Check sheet for the modelled part. Datum: model origin and axes. Units: mm. Face numbers are marked on the shaded views. A direction names the side the tool comes from. Coordinates: 2 decimals unless noted, no trailing zeros. Write each loop counter-clockwise with the first axis right and the second up, starting at its lowest first coordinate (ties: lowest second). Pieces come first, ordered by that corner, then holes. Notation, with made-up numbers: M 85.25,-26.5 L 109.25,-26.5 A35 ccw 109.25,6.5 Z; hole C 88.25,-33 d5. An arc over 180 degrees is marked long. Answer as CSV lines item,"result". Start each with the question number.
Q1. Depth check by flat-ended pin: pin 1 Ø15 at (x, y) = (31.5, -6.5) entering from +Z; pin 2 Ø5 at (y, z) = (-14, 23.5) entering from +X; pin 3 Ø5.5 at (x, z) = (30.5, 9.5) entering from -Y. Enter the tip coordinate at first touch or a pass-through.
Q2. Sectioned sample at B-B, the plane z = 14.5. Record the cut outline in (x, y), then the cut area to 3 significant figures.
Q3. Sectioned sample at C-C, the plane x = 34. Record the cut outline in (y, z).
Q4. Sectioned sample at A-A, the plane y = -9. Record the cut outline in (x, z), then the cut area to 3 significant figures.
Q5. Access from +Z, -Z, +X, -X, +Y, -Y to the whole of each face (thin tool, end or side, straight path). Record for the marked faces 1, 2, 3 and 4.
Q6. Sectioned sample at D-D, the plane x = 16.5. Record the cut outline in (y, z).
Q7. Thickness scan on line 1 along X through (y, z) = (-27.5, 12); line 2 along X through (y, z) = (-17, 25). Record the ranges inside material, lowest first. Write a range as from..to.
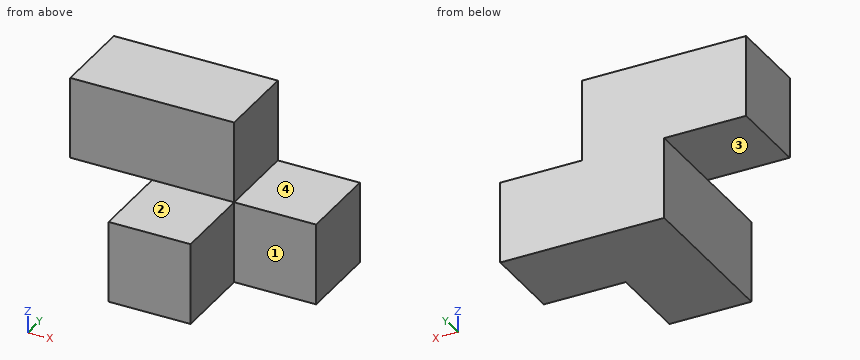
from build123d import *

# Parameters (mm, degrees)
F1_DEPTH = 19.05
F2_W     = 19.05
F2_H     = 19.05
F3_DEPTH = 19.05


with BuildPart() as f1:
    # F0 (on Front) → F1 (new body)
    with BuildSketch(Plane.XZ):
        Polygon((0, 19.05), (0, 0), (38.1, 0), (38.1, 19.05), (19.05, 19.05), (19.05, 38.1), (-19.05, 38.1), (-19.05, 19.05), align=None)
    extrude(amount=F1_DEPTH)

    # F2 (on face) → F3 (join)
    with BuildSketch(Plane.XZ.offset(19.05)):
        with Locations((9.525, 9.525)):
            Rectangle(F2_W, F2_H)
    extrude(amount=F3_DEPTH)


solid = f1.part
Output:
1,pin 1,"stops at z = 19.05"
1,pin 2,"stops at x = 19.05"
1,pin 3,"stops at y = -19.05"
2,outline,"M 0,-38.1 L 19.05,-38.1 L 19.05,-19.05 L 38.1,-19.05 L 38.1,0 L 0,0 Z"
2,area,"1,090 mm^2"
3,outline,"M -19.05,0 L 0,0 L 0,19.05 L -19.05,19.05 Z"
4,outline,"M -19.05,19.05 L 0,19.05 L 0,0 L 38.1,0 L 38.1,19.05 L 19.05,19.05 L 19.05,38.1 L -19.05,38.1 Z"
4,area,"1,450 mm^2"
5,face 1,"+Z, -Z, +X, -Y"
5,face 2,"+Z, +X, -X, -Y"
5,face 3,"-Z, -X, +Y, -Y"
5,face 4,"+Z, +X, +Y, -Y"
6,outline,"M -38.1,0 L 0,0 L 0,38.1 L -19.05,38.1 L -19.05,19.05 L -38.1,19.05 Z"
7,line 1,"x = 0..19.05"
7,line 2,"x = -19.05..19.05"
